```python
from build123d import *

# Parameters (mm, degrees)
F2_T     = -5.08
F4_DEPTH = 38.101
F5_DEPTH = 38.1010001
F6_R     = 0.508


with BuildPart() as f1:
    # F0 (on Front) → F1 (revolve)
    with BuildSketch(Plane.XZ):
        Polygon((0, 0), (0, 63.5), (-38.1, 63.5), (-26.903236725, 0), align=None)
    revolve(axis=Axis((0, 0, 31.75), (0, 0, 1)))

    # F2
    f2_openings = [f1.faces().sort_by_distance(p)[0] for p in [
        (0, 0, 63.5),
    ]]
    offset(amount=F2_T, openings=f2_openings)

    # F3 (on Front) → F4 (cut, through all)
    with BuildSketch(Plane.XZ):
        with BuildLine():
            ThreePointArc((0, 54.61), (-2.6940768363, 48.1059231637), (3.81, 50.8))
            ThreePointArc((3.81, 50.8), (2.6940768363, 53.4940768363), (0, 54.61))
        make_face()
    extrude(amount=F4_DEPTH, mode=Mode.SUBTRACT)

    # F3 (on Front) → F5 (cut, through all)
    with BuildSketch(Plane.XZ):
        with BuildLine():
            ThreePointArc((0, 54.61), (-2.6940768363, 48.1059231637), (3.81, 50.8))
            ThreePointArc((3.81, 50.8), (2.6940768363, 53.4940768363), (0, 54.61))
        make_face()
    extrude(amount=-F5_DEPTH, mode=Mode.SUBTRACT)

    # F6
    f6_edges = [f1.edges().sort_by_distance(p)[0] for p in [
        (38.1, 0, 63.5),
        (32.941633, 0, 63.5),
    ]]
    fillet(f6_edges, radius=F6_R)


solid = f1.part
```
Here's how the part is built. I have some questions about the finished solid (model axes, mm). A direction names the side the tool comes from. Give positions to 0.01 mm unless a question says otherwise; leave off trailing zeros. Write each loop counter-clockwise with the first axis right and the second up, starting at its lowest first coordinate (ties: lowest second). Pieces come first, ordered by that corner, then holes. Notation, with made-up numbers: M -30,-14 L 24,-14 A7 cw 24,-2 Z; hole C -11.5,14.5 d2. An arc over 180 degrees is marked long. Put each result on its own line as item: value. Start each with the question number.
Item 1: If we section it at B-B, the plane x = -2: Count the separate pieces of the cut face and the enclosed holes in it, then the cut area to 3 significant figures.
Item 2: Will these pins go through, and if not, where does the flat tip stop? pin 1 (6 mm diameter, centred on y = -6.5, z = 54, fed in from -X); pin 2 (22.5 mm diameter, centred on x = -9, y = -1.5, fed in from +Z); pin 3 (6 mm diameter, centred on x = -10, z = 48.5, fed in from -Y); pin 4 (6 mm diameter, centred on x = 0, z = 50.8, fed in from +Y).
Item 3: On a 3-axis mill with a long thin cutter (end or side, diameter ignored), from which of +Z, -Z, +X, -X, +Y, -Y can I reach the whole of each face in a straight line? I mean faces 1 (the flat face through (0, 0, 5.08)), 2 (the flat face through (0, 0, 0)). Say none if no direction works.
Item 4: Thinking about a two-plate mould opening in X: for faces 3 (the flat face through (-34, 3, 63.5)), 4 (the conical face through (5.8, 25.9, 27.2)), 5 (the conical face through (6.75, 30.4, 24.02)), which applies, +X half, -X half, draft (parallel to the pull), parting line (faces both ways), or undercut?
Item 5: If we section it at A-A, the plane y = 0: Write out the boundary of the cut face in (x, z).
Item 6: If we section it at C-C, the plane z = 38.5: Write out the boundary of the cut face in (x, y), then the cut area to 3 significant figures.
Item 7: If we section it at D-D, the plane z = 10: Write out the boundary of the cut face in (x, y), then the cut area to 3 significant figures.
Item 8: I need wall thicknesses on L1, parallel to X at y = -31.5, z = 50.8; L2, parallel to Z at x = 4.5, y = -4; L3, parallel to Y at x = -7, z = 34. Which ranges of each line are inside material? Lowest first, please. Write a range as from..to.
Values:
1. separate pieces: 3
1. enclosed holes: 0
1. area: 814 mm²
2. pin 1: x = -36.55
2. pin 2: z = 5.08
2. pin 3: y = -34.96
2. pin 4: through
3. face 1: +Z
3. face 2: -Z, +X, -X, +Y, -Y
4. face 3: draft
4. face 4: undercut
4. face 5: parting line
5. outline: M -37.99,62.9 L -26.9,0 L 26.9,0 L 37.99,62.9 A0.51 ccw 37.49,63.5 L 33.37,63.5 A0.51 ccw 32.87,63.08 L 22.64,5.08 L -22.64,5.08 L -32.87,63.08 A0.51 ccw -33.37,63.5 L -37.49,63.5 A0.51 ccw Z
6. outline: C 0,0 d67.38; hole C 0,0 d57.07
6. area: 1,010 mm²
7. outline: C 0,0 d57.33; hole C 0,0 d47.02
7. area: 846 mm²
8. L1: -17.14..-3.81, 3.81..17.14
8. L2: 0..5.08
8. L3: -32.15..-26.84, 26.84..32.15
